Source: CAD feature listing. Evaluate the final solid. Frame: model axes, mm. Face numbers are marked on the shaded views. A direction names the side the tool comes from. Give positions to 0.01 mm unless a question says otherwise; leave off trailing zeros. Order: outer loops, then holes, each group sorted by start corner. A loop starts at its lowest first (then second) coordinate and runs counter-clockwise, first axis right, second up.
Autodesk Inventor part; units mm, degrees
ref_plane "Plano de trabajo1" through (0, 4.5, 0) normal (0, 1, 0) x (1, 0, 0)
ref_plane "YZ Plane" through (0, 0, 0) normal (1, 0, 0) x (0, 1, 0)
ref_plane "XZ Plane" through (0, 0, 0) normal (0, 1, 0) x (-1, 0, 0)
sketch "Boceto1" plane through (0, 0, 0) normal (0, 1, 0) x (-1, 0, 0)
  circle A0 centre (0, 0) radius 4
  circle A1 centre (0, 0) radius 1
  dimension "d0" = 8
  dimension "d7" = 2
extrude "Extrusión1" add sketch "Boceto1" along normal mid plane 12
ref_plane "Plano de trabajo1" through (0, 4.5, 0) normal (0, 1, 0) x (1, 0, 0)
sketch "Boceto2" plane through (0, 4.5, 0) normal (0, 1, 0) x (1, 0, 0)
  circle A0 centre (0, 0) radius 4
  circle A1 centre (0, 0) radius 2.9
  dimension "d4" = 5.8
extrude "Extrusión2" cut sketch "Boceto2" against normal blind 1.5
mirror "Simetría1" about plane through (0, 0, 0) normal (0, 1, 0) of "Extrusión2"
properties part number "antivibracion_3DPrint"
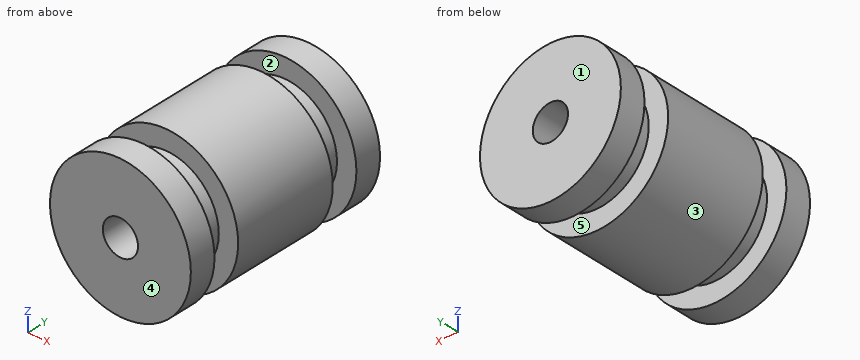
1) Section query A-A, the plane z = 0. Return the cut outline in (x, y), and give its area (3 significant figures).
Report:
outline: (-4, -6) - (-1, -6) - (-1, 6) - (-4, 6) - (-4, 4.5) - (-2.9, 4.5) - (-2.9, 3) - (-4, 3) - (-4, -3) - (-2.9, -3) - (-2.9, -4.5) - (-4, -4.5) - close; (1, -6) - (4, -6) - (4, -4.5) - (2.9, -4.5) - (2.9, -3) - (4, -3) - (4, 3) - (2.9, 3) - (2.9, 4.5) - (4, 4.5) - (4, 6) - (1, 6) - close
area: 65.4 mm2
2) Material intervals for L1, parallel to Y at x = 1.5, z = 2.75; L2, parallel to Z at x = 0, y = 1.25; L3, parallel to X at y = 1, z = 2.75, sorted ascending.
Report:
L1: y = -6 to -4.5, -3 to 3, 4.5 to 6
L2: z = -4 to -1, 1 to 4
L3: x = -2.9 to 2.9
3) Section query B-B, the plane x = 0. Return the cut outline in (y, z).
Report:
outline: (-6, -4) - (-4.5, -4) - (-4.5, -2.9) - (-3, -2.9) - (-3, -4) - (3, -4) - (3, -2.9) - (4.5, -2.9) - (4.5, -4) - (6, -4) - (6, -1) - (-6, -1) - close; (-6, 1) - (6, 1) - (6, 4) - (4.5, 4) - (4.5, 2.9) - (3, 2.9) - (3, 4) - (-3, 4) - (-3, 2.9) - (-4.5, 2.9) - (-4.5, 4) - (-6, 4) - close
4) Pin query (flat end, axial travel): pin 1 (1.5 mm diameter, centred on x = -1.5, y = 4, fed in from +Z); pin 2 (1.5 mm diameter, centred on y = 1.5, z = 3, fed in from +X); pin 3 (1.5 mm diameter, centred on x = 2.5, y = 4, fed in from -Z). Return the tip coordinate at first contact, or that it passes through.
Report:
pin 1: stops at z = 3.89
pin 2: stops at x = 3.31
pin 3: stops at z = -3.5
5) Section query C-C, the plane z = -1.5. Return the cut outline in (x, y).
Report:
outline: (-3.71, -6) - (3.71, -6) - (3.71, -4.5) - (2.48, -4.5) - (2.48, -3) - (3.71, -3) - (3.71, 3) - (2.48, 3) - (2.48, 4.5) - (3.71, 4.5) - (3.71, 6) - (-3.71, 6) - (-3.71, 4.5) - (-2.48, 4.5) - (-2.48, 3) - (-3.71, 3) - (-3.71, -3) - (-2.48, -3) - (-2.48, -4.5) - (-3.71, -4.5) - close
6) Section query D-D, the plane x = 1.5. Return the cut outline in (y, z), and give its area (3 significant figures).
Report:
outline: (-6, -3.71) - (-4.5, -3.71) - (-4.5, -2.48) - (-3, -2.48) - (-3, -3.71) - (3, -3.71) - (3, -2.48) - (4.5, -2.48) - (4.5, -3.71) - (6, -3.71) - (6, 3.71) - (4.5, 3.71) - (4.5, 2.48) - (3, 2.48) - (3, 3.71) - (-3, 3.71) - (-3, 2.48) - (-4.5, 2.48) - (-4.5, 3.71) - (-6, 3.71) - close
area: 81.6 mm2
7) Reachability of the marked faces 4 and 5 from +Z, -Z, +X, -X, +Y, -Y: full face, straight path, thin tool, end or side. Return the list, or none.
Report:
face 4: +Z, -Z, +X, -X, -Y
face 5: none
8) Draft query along Y for the marked faces 1, 2 and 3. Return one class per face: +Y half, -Y half, draft (parallel to the pull), parting line (faces both ways), or undercut.
Report:
face 1: +Y half
face 2: undercut
face 3: draft
